Design review of the part built by this model. Coordinates are the model's own, in mm. A direction names the side the tool comes from. Give positions to 0.01 mm unless a question says otherwise; leave off trailing zeros. Order: outer loops, then holes, each group sorted by start corner. A loop starts at its lowest first (then second) coordinate and runs counter-clockwise, first axis right, second up. Notation, with made-up numbers: (-2, -10) -> (5, -10) arc R22 cw to (5, 15) -> close; hole circle Ø2 at (-19, 8.5). An arc over 180 degrees is marked (long way). One line per item, written item: value.
from build123d import *

# Parameters (mm, degrees)
F5_DEPTH = 5
F7_DEPTH = 2


with BuildPart() as f3:
    # F2 (on Front) → F3 (revolve)
    with BuildSketch(Plane.XZ):
        Polygon((1055, 0), (0, 0), (0, -17.5), (62, -17.5), (62, -20), (120, -20), (120, -25), (1003, -25), (1003, -20), (1055, -20), align=None)
    revolve(axis=Axis((527.5, 0, 0), (1, 0, 0)))

    # F4 (on offset) → F5 (cut)
    with BuildSketch(Plane.XZ.offset(17.5)):
        with BuildLine():
            Line((55, 5), (0, 5))
            Line((0, 5), (0, -5))
            Line((0, -5), (55, -5))
            ThreePointArc((55, -5), (60, 0), (55, 5))
        make_face()
    extrude(amount=-F5_DEPTH, mode=Mode.SUBTRACT)

    # F6 (on offset) → F7 (cut)
    with BuildSketch(Plane.XZ.offset(25)):
        with BuildLine():
            Line((993, 5), (130, 5))
            ThreePointArc((130, 5), (125, 0), (130, -5))
            Line((130, -5), (993, -5))
            ThreePointArc((993, -5), (998, 0), (993, 5))
        make_face()
    extrude(amount=-F7_DEPTH, mode=Mode.SUBTRACT)


solid = f3.part
Item 1: Clearance check with flat-ended pins moving along their axes: P1, Ø10, axis at x = 854.5, y = 11.5, coming from the -Z side; P2, Ø1, axis at x = 301, y = 19.5, coming from the +Z side; P3, Ø6, axis at x = 465.5, y = 15, coming from the -Z side. State where each tip first meets the part, or that it passes through.
Returned:
P1: z = -24.14
P2: z = 16.25
P3: z = -21.93
Item 2: To check wall thickness, follow line 1 along X through (y, z) = (-18, -1); line 2 along X through (y, z) = (19.5, -5); line 3 along Z through (x, y) = (641, -0.5) (3 decimals). State the ranges of each line that lie inside material, in increasing order. Write a range as from..to.
Returned:
line 1: 62..1055
line 2: 120..1003
line 3: -24.995..24.995
Item 3: Add section B-B on x = 606.5. Give the boundary of the cut face in (y, z).
Returned:
outline: (-24.49, -5) arc R25 ccw (long way) to (-24.49, 5) -> (-23, 5) -> (-23, -5) -> close
Item 4: Machinability: for faces 1 (the cylindrical face through (567.681, 7.509, -23.846)), 2 (the cylindrical face through (31.434, 14.756, -9.408)), 3 (the cylindrical face through (1029.364, -19.524, 4.336)), which of the approach directions +Z, -Z, +X, -X, +Y, -Y give a long, thin tool a straight path to every point of the face, cutting with its end or side? Answer none if there is none.
Returned:
face 1: +X, -X
face 2: -X
face 3: +X
Item 5: Add section A-A on y = 0. Give the boundary of the cut face in (x, z), plus the area to 3 significant figures.
Returned:
outline: (0, -17.5) -> (62, -17.5) -> (62, -20) -> (120, -20) -> (120, -25) -> (1003, -25) -> (1003, -20) -> (1055, -20) -> (1055, 20) -> (1003, 20) -> (1003, 25) -> (120, 25) -> (120, 20) -> (62, 20) -> (62, 17.5) -> (0, 17.5) -> close
area: 50,700 mm²
